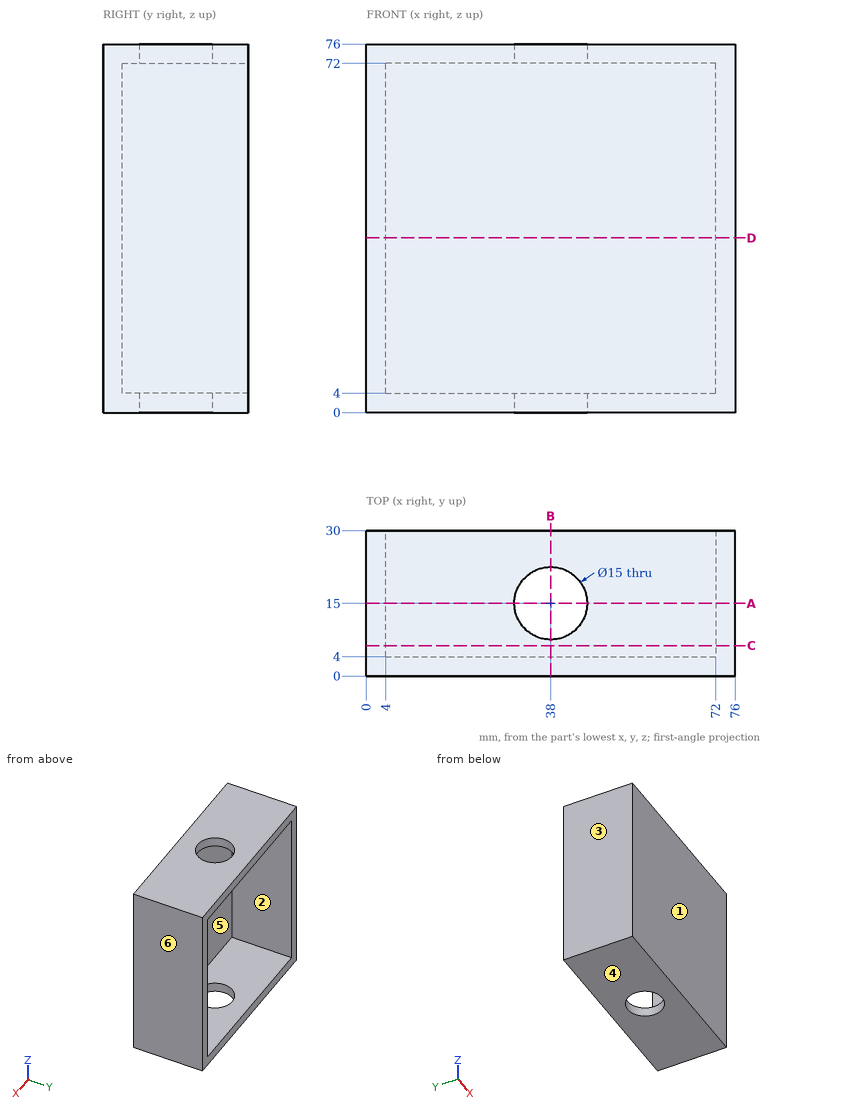
Geometry check sheet. Reference: drawing and pictorial views, mm from the part's lowest x, y, z. A direction names the side the tool comes from. Give positions to 0.01 mm unless a question says otherwise; leave off trailing zeros. Loops run counter-clockwise (first coordinate to the right, second up) from the corner with the lowest first, then second, coordinate; pieces in that order, holes last.
1. Section check B-B, the plane x = 38. Enter the section's corners in (y, z).
2. Mould release check, pull along X, two halves, no side actions. Record for the marked faces 3, 4, 5 and 6: released by +X, released by -X, zero draft, split by the parting line, or undercut.
3. Thickness scan on line 1 (X direction, y = 11, z = 42.5); line 2 (Y direction, x = 38, z = 2). Record the ranges inside material, lowest first.
4. Section check C-C, the plane y = 6.25. Enter the section's corners in (x, z), then the cut area to 3 significant figures.
5. Section check A-A, the plane y = 15. Enter the section's corners in (x, z), then the cut area to 3 significant figures.
6. Set-up check for the marked faces 1 and 2: record each of +Z, -Z, +X, -X, +Y, -Y from which the full face is reachable in a straight line by a thin tool's end or side.
7. Section check D-D, the plane z = 36. Enter the section's corners in (x, y).
8. Go/stop test with a flat-tipped pin: pin 1 Ø8 at (x, z) = (27.5, 47) entering from +Y. Record where the tip stops, or that it passes through.
Geometry says:
1. outline: (0, 0) - (7.5, 0) - (7.5, 4) - (4, 4) - (4, 72) - (7.5, 72) - (7.5, 76) - (0, 76) - close; (22.5, 0) - (30, 0) - (30, 4) - (22.5, 4) - close; (22.5, 72) - (30, 72) - (30, 76) - (22.5, 76) - close
2. face 3: released by -X
2. face 4: zero draft
2. face 5: undercut
2. face 6: released by +X
3. line 1: x = 0 to 4, 72 to 76
3. line 2: y = 0 to 7.5, 22.5 to 30
4. outline: (0, 0) - (76, 0) - (76, 76) - (0, 76) - close; hole (4, 4) - (72, 4) - (72, 72) - (4, 72) - close
4. area: 1,150 mm2
5. outline: (0, 0) - (30.5, 0) - (30.5, 4) - (4, 4) - (4, 72) - (30.5, 72) - (30.5, 76) - (0, 76) - close; (45.5, 0) - (76, 0) - (76, 76) - (45.5, 76) - (45.5, 72) - (72, 72) - (72, 4) - (45.5, 4) - close
5. area: 1,030 mm2
6. face 1: +Z, -Z, +X, -X, -Y
6. face 2: +Y
7. outline: (0, 0) - (76, 0) - (76, 30) - (72, 30) - (72, 4) - (4, 4) - (4, 30) - (0, 30) - close
8. pin 1: stops at y = 4
